Autodesk Inventor part; units mm, degrees
ref_plane "YZ Plane" through (0, 0, 0) normal (1, 0, 0) x (0, 1, 0)
ref_plane "XZ Plane" through (0, 0, 0) normal (0, 1, 0) x (-1, 0, 0)
ref_plane "XY Plane" through (0, 0, 0) normal (0, 0, 1) x (1, 0, 0)
sketch "Sketch1" plane through (0, 0, 0) normal (0, 0, 1) x (1, 0, 0)
  line L0 (0, 0) -> (220, 0)
  line L1 (220, 0) -> (220, 250)
  line L2 (220, 250) -> (0, 250)
  line L3 (0, 250) -> (0, 0)
  dimension "d0" = 220
  dimension "d1" = 250
extrude "Extrusion1" add sketch "Sketch1" along normal blind 100
sketch "Sketch2" plane through (0, 0, 0) normal (0, 0, 1) x (1, 0, 0)
  line L0 (5, 5) -> (215, 5)
  line L1 (215, 5) -> (215, 245)
  line L2 (215, 245) -> (5, 245)
  line L3 (5, 245) -> (5, 5)
  point P0 (0, 0)
  dimension "d4" = 210
  dimension "d5" = 240
  dimension "d8" = 5
  dimension "d13" = 5
extrude "Extrusion2" cut sketch "Sketch2" along normal blind 95
sketch "Sketch3" plane through (220, 0, 0) normal (1, 0, 0) x (0, 0, -1)
  circle A0 centre (-23.8569, 230) radius 15
  line L0 (0, 250) -> (-100, 250)
  point P0 (0, 0)
  dimension "d9" = 30
  dimension "d10" = 20
extrude "Extrusion3" cut sketch "Sketch3" against normal blind 45
sketch "Sketch4" plane through (0, 0, 0) normal (-1, 0, 0) x (0, 0, 1)
  circle A0 centre (73.7116, 232.2043) radius 14.7089
  point P0 (0, 0)
extrude "Extrusion4" cut sketch "Sketch4" against normal blind 10
properties part number "corpo"
CAD build for the part. Positions are in the model's coordinates, mm. A direction names the side the tool comes from. Round coordinates to 2 decimals unless told otherwise and drop trailing zeros. Write each loop counter-clockwise with the first axis right and the second up, starting at its lowest first coordinate (ties: lowest second). Pieces come first, ordered by that corner, then holes.
(1) Slice it at B-B, the plane x = 95. Write the cut outline in (y, z).
(2) Drop a flat-ended pin along its axis: P1, Ø8, axis at x = 105.5, y = 31.5, coming from the -Z side. Give the stop position or say it passes through.
(3) Mould opens along Z. For faces 4 (the face through (108, 0, 49)), 5 (the face through (2.71, 246.79, 71.8)), 6 (the face through (108, 127, 100)) say: pulls with the +Z half, pulls with the -Z half, needs draft (parallel to the pull), parting line crosses it, or undercut.
(4) Slice it at C-C, the plane y = 94. Write the cut outline in (x, z).
(5) Slice it at D-D, the plane z = 84.5. Write the cut outline in (x, y).
(6) 3-axis set-ups, long thin cutter, end or side, ignore diameter. For faces 1 (the face through (217.535, 215.357, 27.109)), 2 (the face through (111, 245, 47)), 3 (the face through (220, 123, 49)): which of +Z, -Z, +X, -X, +Y, -Y reach the whole face in a straight line?
(7) Probe line 1 along Y through (x, z) = (204, 20); line 2 along X through (y, z) = (47.5, 58.5); line 3 along Z through (x, y) = (217, 230). List the from-to ranges inside material, lowest first.
(8) Slice it at A-A, the plane z = 54. Write the cut outline in (x, y), and give its area (3 significant figures).
From the geometry:
1. outline: (0, 0) - (5, 0) - (5, 95) - (245, 95) - (245, 0) - (250, 0) - (250, 100) - (0, 100) - close
2. P1: stops at z = 95
3. face 4: needs draft
3. face 5: undercut
3. face 6: pulls with the +Z half
4. outline: (0, 0) - (5, 0) - (5, 95) - (215, 95) - (215, 0) - (220, 0) - (220, 100) - (0, 100) - close
5. outline: (0, 0) - (220, 0) - (220, 250) - (0, 250) - (0, 242.2) - (5, 242.2) - (5, 245) - (215, 245) - (215, 5) - (5, 5) - (5, 222.21) - (0, 222.21) - close
6. face 1: +X
6. face 2: -Z
6. face 3: +Z, -Z, +X, +Y, -Y
7. line 1: y = 0 to 5, 245 to 250
7. line 2: x = 0 to 5, 215 to 220
7. line 3: z = 0 to 8.86, 38.86 to 100
8. outline: (0, 0) - (220, 0) - (220, 250) - (0, 250) - close; hole (5, 5) - (215, 5) - (215, 245) - (5, 245) - close
8. area: 4,600 mm2
